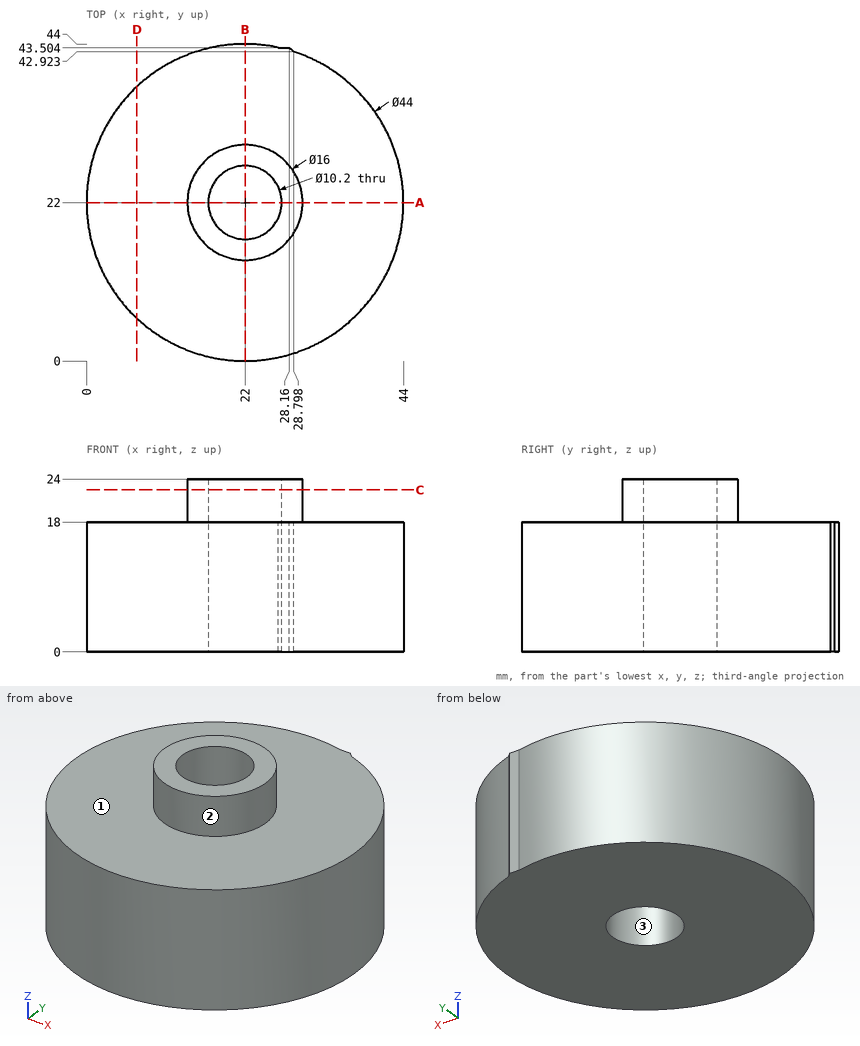
Geometry: see drawing. Coordinates: mm, zero at the bounding-box minimum. Round coordinates to 2 decimals unless told otherwise and drop trailing zeros. Loops run counter-clockwise (first coordinate to the right, second up) from the corner with the lowest first, then second, coordinate; pieces in that order, holes last. Notation, with made-up numbers: (82.25, 80.25) - (89.25, 80.25) arc R29 cw to (89.25, 100.25) - close; hole circle Ø6 at (39.5, 66). An arc over 180 degrees is marked (long way). Write item = value, one per line. Start each with the question number.
(1) Section query D-D, the plane x = 7. Output: boundary loops of the cut face in (y, z), plus the area to 3 significant figures.
(2) Section query C-C, the plane z = 22.5. Output: boundary loops of the cut face in (x, y).
(3) Pin query (flat end, axial travel): pin 1 (6 mm diameter, centred on x = 13, z = 21.5, fed in from -Y); pin 2 (5 mm diameter, centred on x = 30.5, y = 23, fed in from -Z); pin 3 (10 mm diameter, centred on x = 34, z = 2.5, fed in from -Y); pin 4 (4 mm diameter, centred on x = 11, y = 6.5, fed in from +Z). Return the tip coordinate at first contact, or that it passes through.
(4) Pull-direction query (Y, two-part tool) for the marked faces 1, 2 and 3; classes: +Y half, -Y half, draft (parallel to the pull), parting line (faces both ways), or undercut.
(5) Section query A-A, the plane y = 22. Output: boundary loops of the cut face in (x, z), plus the area to 3 significant figures.
(6) Ray query, line 1 along Y through (x, z) = (22, 18.75); line 2 along Z through (x, y) = (8.5, 9); line 3 along Y through (x, z) = (22.5, 1.25) (1 decimal). Return the intervals inside material, ascending. Write a range as from..to.
Conclusion:
q1.outline = (5.91, 0) - (38.09, 0) - (38.09, 18) - (5.91, 18) - close
q1.area = 579 mm2
q2.outline = circle Ø16 at (22, 22); hole circle Ø10.2 at (22, 22)
q3.pin_1 = 16.71
q3.pin_2 = 0
q3.pin_3 = 1.14
q3.pin_4 = 18
q4.face_1 = draft
q4.face_2 = parting line
q4.face_3 = undercut
q5.outline = (0, 0) - (16.9, 0) - (16.9, 24) - (14, 24) - (14, 18) - (0, 18) - close; (27.1, 0) - (44, 0) - (44, 18) - (30, 18) - (30, 24) - (27.1, 24) - close
q5.area = 643 mm2
q6.line_1 = 14..16.9, 27.1..30
q6.line_2 = 0..18
q6.line_3 = 0..16.9, 27.1..44
